Here's how the part is built. I have some questions about the finished solid (model axes, mm). Face numbers are marked on the shaded views. A direction names the side the tool comes from. Round coordinates to 2 decimals unless told otherwise and drop trailing zeros. Write each loop counter-clockwise with the first axis right and the second up, starting at its lowest first coordinate (ties: lowest second). Pieces come first, ordered by that corner, then holes. Notation, with made-up numbers: M 29.5,89.5 L 35.5,89.5 A14 cw 35.5,100.5 Z; hole C 4.25,14.5 d10. An arc over 180 degrees is marked long. Use a Markdown table: item, result. Add a question column.
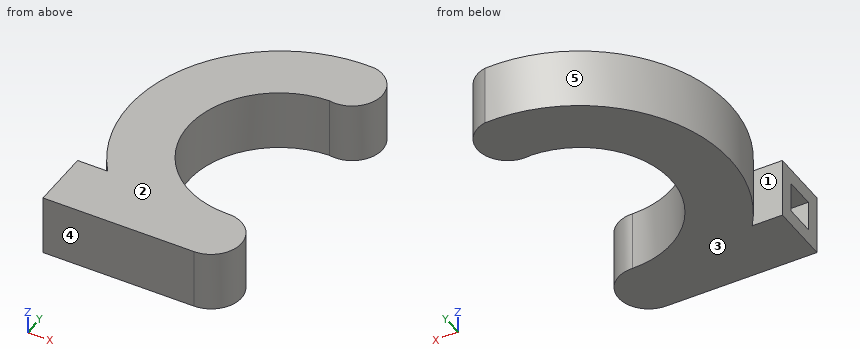
```python
from build123d import *

# Parameters (mm, degrees)
PAD_DEPTH    = 4
SKETCH001_W  = 2
SKETCH001_H  = 2
POCKET_DEPTH = 10


with BuildPart() as part:
    # Sketch → Pad (new body)
    with BuildSketch(Plane.XY):
        with BuildLine():
            Line((2, 4), (0, 4))
            Line((0, 4), (0, 0))
            Line((0, 0), (10, 0))
            ThreePointArc((10, 0), (11.999695, 2.034905), (9.930201, 3.998782))
            ThreePointArc((9.8035, 15.997444), (3.930535, 9.935427), (9.930201, 3.998782))
            ThreePointArc((9.8035, 15.997444), (12.157765, 17.565064), (10.590145, 19.91933))
            ThreePointArc((10.590145, 19.91933), (1.248586, 14.682773), (2, 4))
        make_face()
    extrude(amount=PAD_DEPTH)

    # Sketch001 (on DatumPlane) → Pocket (cut)
    with BuildSketch(Plane(origin=(0, 0, 0), x_dir=(0, -1, 0), z_dir=(-1, 0, 0))):
        with Locations((-2.001803, 1.992215)):
            Rectangle(SKETCH001_W, SKETCH001_H)
    extrude(amount=-POCKET_DEPTH, mode=Mode.SUBTRACT)


solid = part.part
```
Item 1: Imagine slicing it at A-A on x = 1. List the corners of the cut face in (y, z) for me, plus the area to 3 significant figures.
Item 2: Imagine slicing it at D-D on x = 3.5. List the corners of the cut face in (y, z) for me.
Item 3: Imagine slicing it at B-B on y = 2. List the corners of the cut face in (x, z) for me, plus the area to 3 significant figures.
Item 4: On a 3-axis mill with a long thin cutter (end or side, diameter ignored), from which of +Z, -Z, +X, -X, +Y, -Y can I reach the whole of each face in a straight line? I mean the marked faces 1 and 2. Say none if no direction works.
Item 5: I need wall thicknesses on probe 1 along Y at (x, z) = (9.75, 1.6); probe 2 along Y at (x, z) = (8, 1.35); probe 3 along Y at (x, z) = (1.25, 0.6). Which ranges of each line are inside material? Lowest first, please. Write a range as from..to.
Item 6: For pin 1 Ø2 at (x, z) = (2.5, 1.5) entering from +Y; pin 2 Ø1 at (x, z) = (1, 2) entering from +Y; pin 3 Ø1.5 at (y, z) = (3, 1.5) entering from +X; pin 4 Ø1 at (x, y) = (6, 2) entering from -Z, each with a flat end and sliding along its axis, tell me the tip position at first contact or that it passes through.
Item 7: If we mould it in two halves opening along Y, with no side actions, what happens to the marked faces 3, 4 and 5? For each: +Y half, -Y half, draft (parallel to the pull), parting line (faces both ways), or undercut.
The answers:
| question | item | result |
|---|---|---|
| 1 | outline | M 0,0 L 4,0 L 4,4 L 0,4 Z; M 5.68,0 L 14.19,0 L 14.19,4 L 5.68,4 Z; hole M 1,0.99 L 3,0.99 L 3,2.99 L 1,2.99 Z |
| 1 | area | 46.0 mm² |
| 2 | outline | M 0,0 L 17.49,0 L 17.49,4 L 0,4 Z; hole M 1,0.99 L 3,0.99 L 3,2.99 L 1,2.99 Z |
| 3 | outline | M 0,0 L 12,0 L 12,4 L 0,4 L 0,2.99 L 10,2.99 L 10,0.99 L 0,0.99 Z |
| 3 | area | 28.0 mm² |
| 4 | face 1 | +Z, -Z, -X |
| 4 | face 2 | +Z, +X, -X, +Y, -Y |
| 5 | probe 1 | 0..1, 3..4, 16..19.93 |
| 5 | probe 2 | 0..1, 3..4.32, 15.68..19.72 |
| 5 | probe 3 | 0..4, 5.18..14.69 |
| 6 | pin 1 | y = 17.49 |
| 6 | pin 2 | y = 15.12 |
| 6 | pin 3 | x = 11.98 |
| 6 | pin 4 | z = 0 |
| 7 | face 3 | draft |
| 7 | face 4 | -Y half |
| 7 | face 5 | undercut |
